from build123d import *

# Parameters (mm, degrees)
BOSS_EXTRUDE1_DEPTH = 6.35
SKETCH2_W           = 19.05
SKETCH2_H           = 101.6
CUT_EXTRUDE2_DEPTH  = 316.541333465
SKETCH3_R           = 4.572
CUT_EXTRUDE3_DEPTH  = 300.006794446


with BuildPart() as part:
    # Sketch1 → Boss-Extrude1 (new body)
    with BuildSketch(Plane(origin=(0, 0, 0), x_dir=(1, 0, 0), z_dir=(0, 1, 0))):
        with BuildLine():
            Line((-257.175, 0), (257.175, 0))
            Line((257.175, 0), (257.175, -104.032493436))
            Line((257.175, -104.032493436), (199.670208733, -104.032493436))
            ThreePointArc((199.670208733, -104.032493436), (107.889594305, -43.469891278), (0, -22.225))
            Line((0, -22.225), (-127, -22.225))
            ThreePointArc((-127, -22.225), (-219.047625241, -60.352374759), (-257.175, -152.4))
            Line((-257.175, -152.4), (-276.225, -152.4))
            Line((-276.225, -152.4), (-276.225, -50.8))
            Line((-276.225, -50.8), (-257.175, -50.8))
            Line((-257.175, -50.8), (-257.175, 0))
        make_face()
    extrude(amount=BOSS_EXTRUDE1_DEPTH)

    # Sketch2 → Cut-Extrude2 (cut, through all)
    with BuildSketch(Plane(origin=(0, 0, 0), x_dir=(1, 0, 0), z_dir=(0, 1, 0))):
        with Locations((-266.7, -101.6)):
            Rectangle(SKETCH2_W, SKETCH2_H)
    extrude(amount=CUT_EXTRUDE2_DEPTH, mode=Mode.SUBTRACT)

    # Sketch3 → Cut-Extrude3 (cut, through all)
    with BuildSketch(Plane(origin=(0, 6.35, 0), x_dir=(1, 0, 0), z_dir=(0, 1, 0))):
        with Locations(Location((-208.452544448, -36.961239505, 0), (0, 0, 270))):
            Circle(SKETCH3_R)
        with Locations(Location((-246.552544448, -36.961239505, 0), (0, 0, 270))):
            Circle(SKETCH3_R)
        with Locations(Location((-231.855506716, -51.658277238, 0), (0, 0, 270))):
            Circle(SKETCH3_R)
        with Locations(Location((-246.552544448, -75.061239505, 0), (0, 0, 270))):
            Circle(SKETCH3_R)
    extrude(amount=-CUT_EXTRUDE3_DEPTH, mode=Mode.SUBTRACT)


solid = part.part
Could you check a few things on this model? Use its own coordinates, in mm. A direction names the side the tool comes from. Coordinates: 2 decimals unless noted, no trailing zeros. Write each loop counter-clockwise with the first axis right and the second up, starting at its lowest first coordinate (ties: lowest second). Pieces come first, ordered by that corner, then holes. Notation, with made-up numbers: (83.25, -37.5) - (94.25, -37.5) arc R5 cw to (94.25, -28.5) - close; hole circle Ø6 at (88.5, 14.5). An arc over 180 degrees is marked (long way). Put each result on its own line as item: value. Start each with the question number.
Q1. I want a section at C-C on z = 108.5. Write out the boundary of the cut face in (x, y) (3 decimals), plus the area to 3 significant figures.
Q2. Please list where these lines run through material, in increasing order: L1, parallel to X at y = 3.75, z = 77.5 (3 decimals); L2, parallel to X at y = 5, z = 78 (3 decimals); L3, parallel to Z at x = -68.5, y = 5.75 (3 decimals).
Q3. I want a section at A-A on y = 2.75. Count the separate pieces of the cut face and the enclosed holes in it, plus the area to 3 significant figures.
Q4. Thinking about a two-plate mould opening in X: for faces 1 (the flat face through (58, 0, 25)), 2 (the cylindrical face through (-251, 3, 74)), which applies, pulls with the +X half, pulls with the -X half, needs draft (parallel to the pull), parting line crosses it, or undercut?
Q5. Which directions (+Z, -Z, +X, -X, +Y, -Y) give clear straight access to the entire face, cutting with the end or side of a thin tool? Please do faces 3 (the cylindrical face through (109.32, 3.13, 44.06)), 4 (the cylindrical face through (-251.016, 3.219, 35.97)).
Q6. I want a section at B-B on x = -112. Write out the boundary of the cut face in (y, z) (3 decimals), plus the area to 3 significant figures.
Q7. I'm going to push flat-ended pins straight in: P1, Ø5.5, axis at x = -246.55, z = 36.96, coming from the +Y side; P2, Ø3, axis at x = -155, y = 2.5, coming from the +Z side; P3, Ø1.9, axis at x = 225, y = 2, coming from the +Z side. Where does each tip first touch, or does it pass through?
Checks:
1. outline: (-257.175, 0) - (-249.549, 0) - (-249.549, 6.35) - (-257.175, 6.35) - close
1. area: 48.4 mm²
2. L1: -257.175 to -250.42, -242.685 to -233.468, 168.536 to 257.175
2. L2: -257.175 to -250.055, -243.05 to -233.818, 169.214 to 257.175
2. L3: 0 to 22.225
3. separate pieces: 1
3. enclosed holes: 4
3. area: 24,600 mm²
4. face 1: needs draft
4. face 2: undercut
5. face 3: +Z, +Y, -Y
5. face 4: +Y, -Y
6. outline: (0, 0) - (6.35, 0) - (6.35, 22.225) - (0, 22.225) - close
6. area: 141 mm²
7. P1: through
7. P2: z = 25.61
7. P3: z = 104.03
